Study the drawing (mm; zero at the part's minimum x, y, z) and answer. Round coordinates to 2 decimals unless told otherwise and drop trailing zeros. Write each loop counter-clockwise with the first axis right and the second up, starting at its lowest first coordinate (ties: lowest second). Pieces come first, ordered by that corner, then holes.
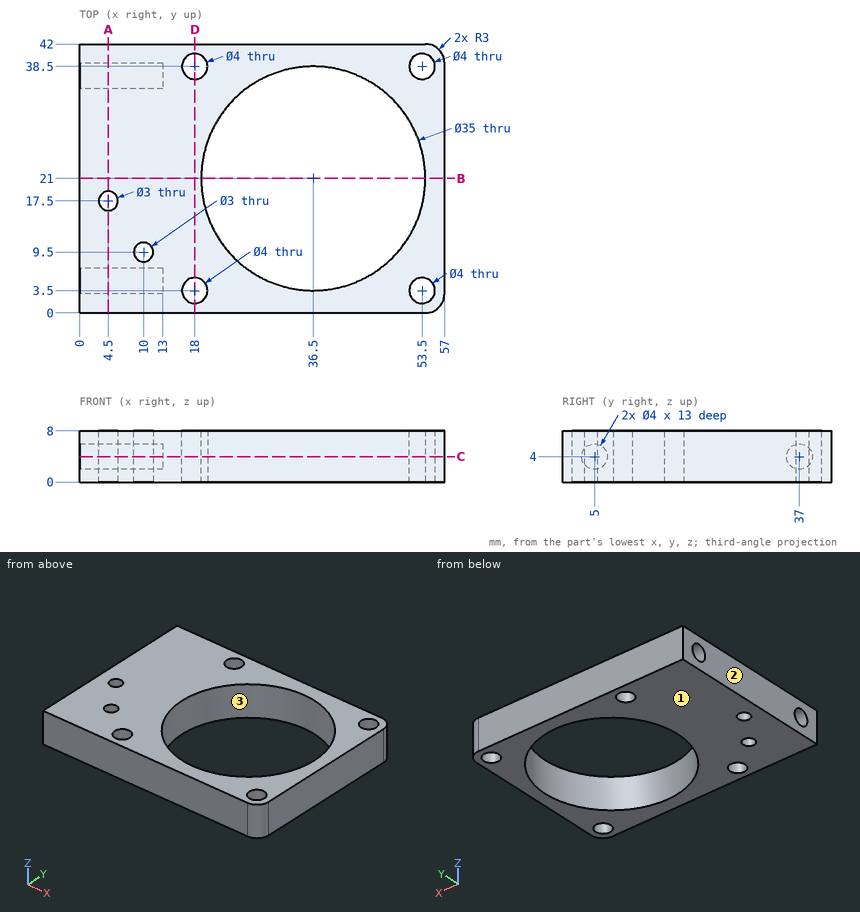
1. Section A-A on x = 4.5 is taken. Determine the outline of the cut face in (y, z).
Geometry says:
outline: (0, 0) - (16, 0) - (16, 8) - (0, 8) - close; (19, 0) - (42, 0) - (42, 8) - (19, 8) - close; hole circle Ø4 at (5, 4); hole circle Ø4 at (37, 4)
2. Section C-C on z = 4 is taken. Determine the outline of the cut face in (x, y).
Geometry says:
outline: (0, 0) - (54, 0) arc R3 ccw to (57, 3) - (57, 39) arc R3 ccw to (54, 42) - (0, 42) - (0, 39) - (13, 39) - (13, 35) - (0, 35) - (0, 7) - (13, 7) - (13, 3) - (0, 3) - close; hole circle Ø3 at (4.5, 17.5); hole circle Ø3 at (10, 9.5); hole circle Ø4 at (18, 3.5); hole circle Ø4 at (18, 38.5); hole circle Ø35 at (36.5, 21); hole circle Ø4 at (53.5, 3.5); hole circle Ø4 at (53.5, 38.5)
3. Section B-B on y = 21 is taken. Determine the outline of the cut face in (x, z).
Geometry says:
outline: (0, 0) - (19, 0) - (19, 8) - (0, 8) - close; (54, 0) - (57, 0) - (57, 8) - (54, 8) - close
4. Straight lines are drawn through the part: line 1 along X through (y, z) = (17, 2.5); line 2 along Y through (x, z) = (18.5, 4.75); line 3 along Y through (x, z) = (52, 7). For each, find the intervals that lie inside material, in ascending order.
Geometry says:
line 1: x = 0 to 3.09, 5.91 to 19.46, 53.54 to 57
line 2: y = 0 to 1.56, 5.44 to 36.56, 40.44 to 42
line 3: y = 0 to 2.18, 4.82 to 12.88, 29.12 to 37.18, 39.82 to 42
5. Section D-D on x = 18 is taken. Determine the outline of the cut face in (y, z).
Geometry says:
outline: (0, 0) - (1.5, 0) - (1.5, 8) - (0, 8) - close; (5.5, 0) - (36.5, 0) - (36.5, 8) - (5.5, 8) - close; (40.5, 0) - (42, 0) - (42, 8) - (40.5, 8) - close
6. For a pull along X with two mould halves and no side action, classify the marked faces 1, 2 and 3 as released by +X, released by -X, zero draft, split by the parting line, or undercut.
Geometry says:
face 1: zero draft
face 2: released by -X
face 3: undercut
7. Given pin 1 (2 mm diameter, centred on y = 37, z = 4, fed in from -X), flat-ended and moving along its own axis, determine where the tip first touches the part or whether it passes through.
Geometry says:
pin 1: stops at x = 13
